Source: CAD feature listing. Evaluate the final solid. Frame: model axes, mm. Face numbers are marked on the shaded views. Round coordinates to 2 decimals unless told otherwise and drop trailing zeros. Loops run counter-clockwise (first coordinate to the right, second up) from the corner with the lowest first, then second, coordinate; pieces in that order, holes last.
(1) Section A-A, the plane z = -4.75. Return the cut outline in (x, y).
(2) Mould query, pull axis X, two halves, no side actions, for the marked faces 1, 2 and 3. Classes: pulls with the +X half, pulls with the -X half, needs draft (parallel to the pull), parting line crosses it, or undercut.
(3) Material intervals for probe 1 along X at (y, z) = (-4.5, -3.5); probe 2 along X at (y, z) = (-2, -1.25); probe 3 along Z at (x, y) = (-0.5, -9.25), sorted ascending.
(4) Section C-C, the plane x = 0. Return the cut outline in (y, z).
(5) Section D-D, the plane z = -1.5. Return the cut outline in (x, y), plus the area to 3 significant figures.
(6) Section B-B, the plane y = -8.5. Return the cut outline in (x, z), plus the area to 3 significant figures.
(7) First-contact query: pin 1 Ø1.5 at (x, z) = (0.5, 2) entering from +Y; pin 2 Ø2 at (x, y) = (-3, -7.5) entering from -Z. Flat tips, straight axial feed; report the tip coordinate or a pass-through.
```python
from build123d import *

# Parameters (mm, degrees)
F1_DEPTH = 12
F2_R     = 2


with BuildPart() as f1:
    # F0 (on Front) → F1 (new body)
    with BuildSketch(Plane.XZ):
        with BuildLine():
            Line((20.25, 6), (-20.25, 6))
            Line((-20.25, 6), (-20.25, -6))
            Line((-20.25, -6), (-4.499552, -6))
            Line((-4.499552, -6), (-4.499552, -3.063528))
            ThreePointArc((-4.499552, -3.063528), (-0.031765, 1.499888), (4.5, -3))
            ThreePointArc((4.5, -3), (4.493441, -3.242866), (4.473785, -3.485024))
            Line((4.473785, -3.485024), (4.473785, -6))
            Line((4.473785, -6), (20.25, -6))
            Line((20.25, -6), (20.25, 6))
        make_face()
    extrude(amount=F1_DEPTH)

    # F2
    f2_edges = [f1.edges().sort_by_distance(p)[0] for p in [
        (20.25, -6, 6),
        (-20.25, -6, 6),
    ]]
    fillet(f2_edges, radius=F2_R)


solid = f1.part
```
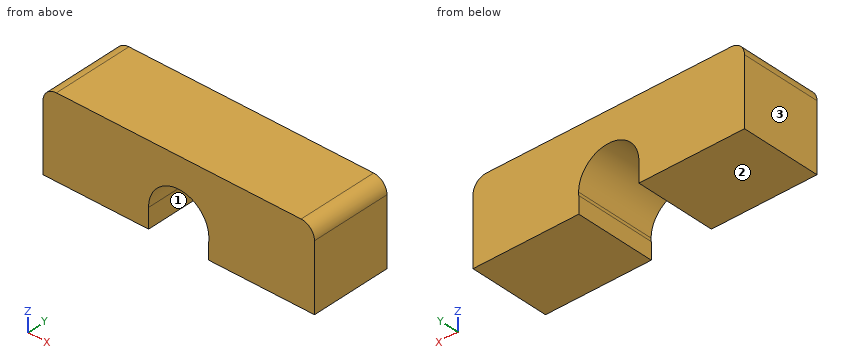
Output values:
1. outline: (-20.25, -12) - (-4.5, -12) - (-4.5, 0) - (-20.25, 0) - close; (4.47, -12) - (20.25, -12) - (20.25, 0) - (4.47, 0) - close
2. face 1: undercut
2. face 2: needs draft
2. face 3: pulls with the -X half
3. probe 1: x = -20.25 to -4.5, 4.47 to 20.25
3. probe 2: x = -20.25 to -4.15, 4.15 to 20.25
3. probe 3: z = 1.47 to 6
4. outline: (-12, 1.5) - (0, 1.5) - (0, 6) - (-12, 6) - close
5. outline: (-20.25, -12) - (-4.24, -12) - (-4.24, 0) - (-20.25, 0) - close; (4.24, -12) - (20.25, -12) - (20.25, 0) - (4.24, 0) - close
5. area: 384 mm2
6. outline: (-20.25, -6) - (-4.5, -6) - (-4.5, -3.06) arc R4.5 cw (long way) to (4.5, -3) arc R4.5 cw to (4.47, -3.49) - (4.47, -6) - (20.25, -6) - (20.25, 4) arc R2 ccw to (18.25, 6) - (-18.25, 6) arc R2 ccw to (-20.25, 4) - close
6. area: 426 mm2
7. pin 1: stops at y = 0
7. pin 2: stops at z = -0.94
